The listing builds one solid part. Answer for the finished solid, in the listing's coordinates (mm). Give positions to 0.01 mm unless a question says otherwise; leave off trailing zeros. Loops run counter-clockwise (first coordinate to the right, second up) from the corner with the lowest first, then second, coordinate; pieces in that order, holes last. Notation, with made-up numbers: (15.25, 56) - (22.25, 56) arc R25 cw to (22.25, 83) - close; hole circle Ø5 at (68.25, 26). An arc over 180 degrees is marked (long way). Write item = value, one per line. Start each with the question number.
1) A flat-ended cylindrical pin translates along its axis: P1, Ø1.5, axis at x = 43.5, y = 65.5, coming from the +Z side. Find the tip coordinate at first contact, or state that the pin passes through.
2) Consider probe 1 along X at (y, z) = (70, 6.75); probe 2 along Y at (x, z) = (30, 20.25); probe 3 along X at (y, z) = (30, 19.25). Determine where each line is inside the solid, lowest interval first.
3) The part is cut by section A-A on y = 70. Write down the section's boundary in (x, z).
4) The part is cut by section C-C on x = 56. Write down the section's boundary in (y, z).
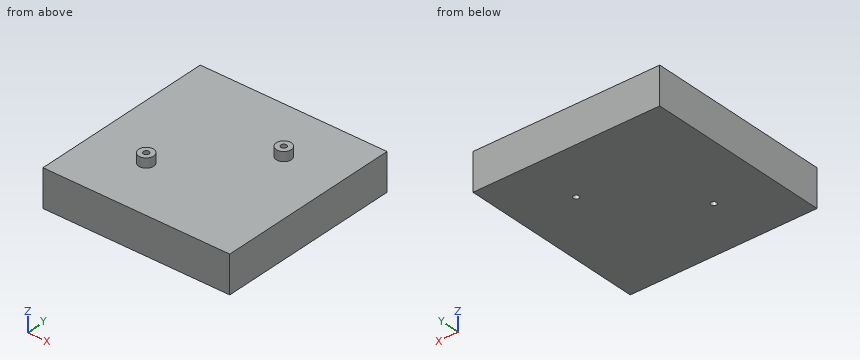
Autodesk Inventor part; units mm, degrees
ref_plane "YZ Plane" through (0, 0, 0) normal (1, 0, 0) x (0, 1, 0)
ref_plane "XZ Plane" through (0, 0, 0) normal (0, 1, 0) x (-1, 0, 0)
ref_plane "XY Plane" through (0, 0, 0) normal (0, 0, 1) x (1, 0, 0)
sketch "Skizze1" plane through (0, 0, 0) normal (0, 0, 1) x (1, 0, 0)
  line L0 (0, 0) -> (100, 0)
  line L1 (100, 0) -> (100, 100)
  line L2 (100, 100) -> (0, 100)
  line L3 (0, 100) -> (0, 0)
  dimension "d0" = 100
  dimension "d1" = 100
extrude "Extrusion1" add sketch "Skizze1" along normal blind 20
sketch "Skizze2" plane through (0, 0, 20) normal (0, 0, 1) x (1, 0, 0)
  line L0 (0, 0) -> (100, 0)
  line L1 (0, 100) -> (0, 0)
  line L2 (100, 100) -> (0, 100)
  line L3 (100, 0) -> (100, 100)
  point P0 (30, 30)
  point P1 (70, 70)
  dimension "d4" = 30
  dimension "d5" = 30
  dimension "d6" = 30
  dimension "d7" = 30
hole "Bohrung1" at (30, 30, 20) at (70, 70, 20) direction (0, 0, -1) diameter 3 end through all
sketch "Skizze3" plane through (0, 0, 20) normal (0, 0, 1) x (1, 0, 0)
  circle A0 centre (30, 30) radius 1.5
  circle A1 centre (30, 30) radius 4
  circle A2 centre (30, 30) radius 1.5
  point P0 (0, 0)
  dimension "d15" = 3
  dimension "d16" = 8
extrude "Extrusion2" add sketch "Skizze3" along normal blind 5
sketch "Skizze4" plane through (0, 0, 20) normal (0, 0, 1) x (1, 0, 0)
  circle A0 centre (70, 70) radius 4
  circle A1 centre (70, 70) radius 1.5
  circle A2 centre (70, 70) radius 1.5
  circle A3 centre (70, 70) radius 1.5
  point P0 (0, 0)
  dimension "d19" = 3
  dimension "d20" = 8
extrude "Extrusion3" add sketch "Skizze4" along normal blind 5
properties part number "platine"
Answer below:
q1.P1 = 20
q2.probe_1 = 0 to 68.5, 71.5 to 100
q2.probe_2 = 26 to 28.5, 31.5 to 34
q2.probe_3 = 0 to 28.5, 31.5 to 100
q3.outline = (0, 0) - (68.5, 0) - (68.5, 25) - (66, 25) - (66, 20) - (0, 20) - close; (71.5, 0) - (100, 0) - (100, 20) - (74, 20) - (74, 25) - (71.5, 25) - close
q4.outline = (0, 0) - (100, 0) - (100, 20) - (0, 20) - close
